from build123d import *

# Parameters (mm, degrees)
SKETCH1_R           = 3.9
BOSS_EXTRUDE1_DEPTH = 16
SKETCH1_3_R         = 4.9
BOSS_EXTRUDE2_DEPTH = 1.5
CUT_EXTRUDE2_START  = 15.9
SKETCH5_R           = 3.9
SKETCH5_R_2         = 2
CUT_EXTRUDE2_DEPTH  = 3.2
CHAMFER1_SIZE       = 1
CHAMFER1_SIZE2      = 0.176326981
BOSS_EXTRUDE3_DEPTH = 0.5
CUT_EXTRUDE1_DEPTH  = 6


with BuildPart() as part:
    # Sketch1 → Boss-Extrude1 (new body)
    with BuildSketch(Plane.XY):
        Circle(SKETCH1_R)
    extrude(amount=-BOSS_EXTRUDE1_DEPTH)

    # Sketch1_3 → Boss-Extrude2 (add)
    with BuildSketch(Plane.XY):
        Circle(SKETCH1_3_R)
    extrude(amount=BOSS_EXTRUDE2_DEPTH)

    # Sketch5 → Cut-Extrude2 (cut)
    with BuildSketch(Plane(origin=(0, 0, 0), x_dir=(-1, 0, 0), z_dir=(0, 0, -1)).offset(CUT_EXTRUDE2_START)):
        with Locations(Location((0, 0, 0), (0, 0, 180))):
            Circle(SKETCH5_R)
        with Locations(Location((0, 0, 0), (0, 0, 180))):
            Circle(SKETCH5_R_2, mode=Mode.SUBTRACT)
    extrude(amount=CUT_EXTRUDE2_DEPTH, mode=Mode.SUBTRACT)

    # Chamfer1
    chamfer1_edges = [part.edges().sort_by_distance(p)[0] for p in [
        (-4.9, 0, 1.5),
    ]]
    chamfer1_side = [part.faces().sort_by_distance(p)[0] for p in [
        (-4.9, 0, 0.75),
    ]]
    chamfer(chamfer1_edges, length=CHAMFER1_SIZE, length2=CHAMFER1_SIZE2, reference=chamfer1_side[0])

    # Sketch2 → Boss-Extrude3 (add)
    with BuildSketch(Plane(origin=(0, 0, -16), x_dir=(-1, 0, 0), z_dir=(0, 0, -1))):
        with BuildLine():
            Line((-3.625126266, 2), (-2.1, 2))
            Line((-2.1, 2), (-2.1, -2))
            Line((-2.1, -2), (-3.625126266, -2))
            Line((-3.625126266, -2), (-3.875126266, -1.75))
            ThreePointArc((-3.875126266, -1.75), (-4.6, 0), (-3.875126266, 1.75))
            Line((-3.875126266, 1.75), (-3.625126266, 2))
        make_face()
    boss_extrude3 = extrude(amount=-BOSS_EXTRUDE3_DEPTH)

    # Sketch4 → Cut-Extrude1 (cut)
    with BuildSketch(Plane(origin=(0, 0, -16), x_dir=(-1, 0, 0), z_dir=(0, 0, -1))):
        Polygon((-3.625126266, -2), (-2.1, -2), (-2.1, 2), (-3.625126266, 2), (-3.625126266, 2.4), (-1.2, 2.4), (-1.2, -2.3), (-3.625126266, -2.3), align=None)
    cut_extrude1 = extrude(amount=-CUT_EXTRUDE1_DEPTH, mode=Mode.SUBTRACT)

    # Mirror1: Boss-Extrude3, Cut-Extrude1 across plane
    add(boss_extrude3.mirror(Plane(origin=(0, 0, 0), x_dir=(0, 0, 1), z_dir=(1, 0, 0))))
    add(cut_extrude1.mirror(Plane(origin=(0, 0, 0), x_dir=(0, 0, 1), z_dir=(1, 0, 0))), mode=Mode.SUBTRACT)


solid = part.part
Work out the finished part from the listing and answer in its coordinate system (mm). A direction names the side the tool comes from. Coordinates: 2 decimals unless noted, no trailing zeros. Write each loop counter-clockwise with the first axis right and the second up, starting at its lowest first coordinate (ties: lowest second). Pieces come first, ordered by that corner, then holes. Notation, with made-up numbers: M -37,43 L -16,43 A23 cw -16,79 Z; hole C -28.5,0 d1. An arc over 180 degrees is marked long. Use one line per item in the form item = value. Start each with the question number.
1. The part is cut by section A-A (z = -12.25). Give the vertices of the cut face in (x, y).
2. The part is cut by section D-D (z = -3). Give the vertices of the cut face in (x, y), plus the area to 3 significant figures.
3. Straight lines are drawn through the part: probe 1 along X at (y, z) = (-1.5, -10.25); probe 2 along Z at (x, y) = (-1.75, 2.75); probe 3 along X at (y, z) = (2.25, -12.5). For each, find the intervals that lie inside material, in ascending order. Write a range as from..to.
4. Each of these flat-tipped pins is pushed along its axis until it touches: P1, Ø4, axis at x = -2, z = -3.5, coming from the +Y side; P2, Ø0.5, axis at x = -3, z = -12, coming from the -Y side; P3, Ø5, axis at y = 0, z = -14, coming from the -X side. Where does it stop, or does it pass through?
5. The part is cut by section C-C (y = 0). Give the vertices of the cut face in (x, z).
6. The part is cut by section B-B (x = 0). Give the vertices of the cut face in (y, z).
7. A tool of negligible diameter and unlimited length cuts with its end or side. For faces 1 (the face through (1.2, 0, -13)), 2 (the face through (-3, -2, -13)), 3 (the face through (-3, 0, -16)), 4 (the face through (3, -2, -13)), 5 (the face through (-1.062, -4.783, 0.246)), from which of +Z, -Z, +X, -X, +Y, -Y can it reach the whole face along a straight path? Write none if from no direction.
8. The mould has two halves that part along Z. Classify faces 6 (the face through (-4.1, 0, -15.5)), 7 (the face through (2, 2.4, -13)), 8 (the face through (3, 0, -16)): released by +Z, released by -Z, zero draft, split by the parting line, or undercut.
Evaluation:
q1.outline = M -3.35,-2 L -2.1,-2 L -2.1,2 L -3.35,2 A3.9 ccw Z; M -3.15,-2.3 A3.9 ccw 3.15,-2.3 L 1.2,-2.3 L 1.2,2.4 L 3.07,2.4 A3.9 ccw -3.07,2.4 L -1.2,2.4 L -1.2,-2.3 Z; M 2.1,-2 L 3.35,-2 A3.9 ccw 3.35,2 L 2.1,2 Z
q2.outline = C 0,0 d7.8
q2.area = 47.8 mm^2
q3.probe_1 = -3.6..-2.1, -1.2..1.2, 2.1..3.6
q3.probe_2 = -15.9..1.5
q3.probe_3 = -1.2..1.2
q4.P1 = 3.9
q4.P2 = -2.77
q4.P3 = -4.6
q5.outline = M -4.9,0 L -3.9,0 L -3.9,-15.5 L -4.6,-15.5 L -4.6,-16 L -2.1,-16 L -2.1,-10 L -1.2,-10 L -1.2,-16 L 1.2,-16 L 1.2,-10 L 2.1,-10 L 2.1,-16 L 4.6,-16 L 4.6,-15.5 L 3.9,-15.5 L 3.9,0 L 4.9,0 L 4.9,0.5 L 4.72,1.5 L -4.72,1.5 L -4.9,0.5 Z
q6.outline = M -4.9,0 L -3.9,0 L -3.9,-15.9 L -2,-15.9 L -2,-16 L 2,-16 L 2,-15.9 L 3.9,-15.9 L 3.9,0 L 4.9,0 L 4.9,0.5 L 4.72,1.5 L -4.72,1.5 L -4.9,0.5 Z
q7.face_1 = -Z
q7.face_2 = -Z, -X
q7.face_3 = -Z, +X, -X, +Y, -Y
q7.face_4 = -Z, +X
q7.face_5 = +Z, -Z
q8.face_6 = undercut
q8.face_7 = zero draft
q8.face_8 = released by -Z
